CAD build for the part. Positions are in the model's coordinates, mm. Round coordinates to 2 decimals unless told otherwise and drop trailing zeros. Loops run counter-clockwise (first coordinate to the right, second up) from the corner with the lowest first, then second, coordinate; pieces in that order, holes last. Notation, with made-up numbers: M -38,57.25 L 12,57.25 A23 ccw 12,89.25 Z; hole C 12,51 d10. An arc over 180 degrees is marked long. Put each result on its own line as item: value. Start each with the question number.
from build123d import *

# Parameters (mm, degrees)
F0_R     = 2.725
F0_R_2   = 10
F0_R_3   = 1
F1_DEPTH = 1.8
F2_DEPTH = 6.3
F3_DEPTH = 6.3
F4_DEPTH = 6.25


with BuildPart() as f1:
    # F0 (on Top) → F1 (new body)
    with BuildSketch(Plane.XY):
        with BuildLine():
            Line((38.875, -34.725), (38.875, 34.725))
            ThreePointArc((38.875, 34.725), (37.659493, 37.659493), (34.725, 38.875))
            Line((34.725, 38.875), (-34.725, 38.875))
            ThreePointArc((-34.725, 38.875), (-37.659493, 37.659493), (-38.875, 34.725))
            Line((-38.875, 34.725), (-38.875, -34.725))
            ThreePointArc((-38.875, -34.725), (-37.659493, -37.659493), (-34.725, -38.875))
            Line((-34.725, -38.875), (34.725, -38.875))
            ThreePointArc((34.725, -38.875), (37.659493, -37.659493), (38.875, -34.725))
        make_face()
        with Locations((-22.925, -34.725)):
            Circle(F0_R, mode=Mode.SUBTRACT)
        with Locations((22.925, -34.725)):
            Circle(F0_R, mode=Mode.SUBTRACT)
        with Locations((-22.925, 34.725)):
            Circle(F0_R, mode=Mode.SUBTRACT)
        Circle(F0_R_2, mode=Mode.SUBTRACT)
        with Locations((22.925, 34.725)):
            Circle(F0_R, mode=Mode.SUBTRACT)
        with Locations((-22.925, 34.725)):
            Circle(F0_R)
        with Locations((-22.925, 34.725)):
            Circle(F0_R_3, mode=Mode.SUBTRACT)
        with Locations((-22.925, 34.725)):
            Circle(F0_R_3)
        with Locations((22.925, -34.725)):
            Circle(F0_R)
        with Locations((22.925, -34.725)):
            Circle(F0_R_3, mode=Mode.SUBTRACT)
        with Locations((22.925, -34.725)):
            Circle(F0_R_3)
        with Locations((-22.925, -34.725)):
            Circle(F0_R)
        with Locations((-22.925, -34.725)):
            Circle(F0_R_3, mode=Mode.SUBTRACT)
        with Locations((-22.925, -34.725)):
            Circle(F0_R_3)
        with Locations((22.925, 34.725)):
            Circle(F0_R)
        with Locations((22.925, 34.725)):
            Circle(F0_R_3, mode=Mode.SUBTRACT)
        with Locations((22.925, 34.725)):
            Circle(F0_R_3)
    extrude(amount=F1_DEPTH)

    # F0 (on Top) → F2 (join)
    with BuildSketch(Plane.XY):
        with BuildLine():
            Line((-34.725, -40.725), (34.725, -40.725))
            ThreePointArc((34.725, -40.725), (38.967641, -38.967641), (40.725, -34.725))
            Line((40.725, -34.725), (40.725, 34.725))
            ThreePointArc((40.725, 34.725), (38.967641, 38.967641), (34.725, 40.725))
            Line((34.725, 40.725), (-34.725, 40.725))
            ThreePointArc((-34.725, 40.725), (-38.967641, 38.967641), (-40.725, 34.725))
            Line((-40.725, 34.725), (-40.725, -34.725))
            ThreePointArc((-40.725, -34.725), (-38.967641, -38.967641), (-34.725, -40.725))
        make_face()
        with BuildLine():
            ThreePointArc((34.725, 38.875), (37.659493, 37.659493), (38.875, 34.725))
            Line((38.875, 34.725), (38.875, -34.725))
            ThreePointArc((38.875, -34.725), (37.659493, -37.659493), (34.725, -38.875))
            Line((34.725, -38.875), (-34.725, -38.875))
            ThreePointArc((-34.725, -38.875), (-37.659493, -37.659493), (-38.875, -34.725))
            Line((-38.875, -34.725), (-38.875, 34.725))
            ThreePointArc((-38.875, 34.725), (-37.659493, 37.659493), (-34.725, 38.875))
            Line((-34.725, 38.875), (34.725, 38.875))
        make_face(mode=Mode.SUBTRACT)
    extrude(amount=F2_DEPTH)

    # F0 (on Top) → F3 (join)
    with BuildSketch(Plane.XY):
        with Locations((-22.925, 34.725)):
            Circle(F0_R)
        with Locations((-22.925, 34.725)):
            Circle(F0_R_3, mode=Mode.SUBTRACT)
    extrude(amount=F3_DEPTH)

    # F0 (on Top) → F4 (join)
    with BuildSketch(Plane.XY):
        with Locations((22.925, 34.725)):
            Circle(F0_R)
        with Locations((22.925, 34.725)):
            Circle(F0_R_3, mode=Mode.SUBTRACT)
        with Locations((22.925, -34.725)):
            Circle(F0_R)
        with Locations((22.925, -34.725)):
            Circle(F0_R_3, mode=Mode.SUBTRACT)
        with Locations((-22.925, -34.725)):
            Circle(F0_R)
        with Locations((-22.925, -34.725)):
            Circle(F0_R_3, mode=Mode.SUBTRACT)
    extrude(amount=F4_DEPTH)


solid = f1.part
(1) Cut at A-A on z = 3.5. Count the separate pieces of the cut face and the enclosed holes in it, and give its area (3 significant figures).
(2) Mould opens along Y. For faces 1 (the cylindrical face through (-23.662, 35.401, 4.018)), 2 (the cylindrical face through (-38.921, 39.014, 3.106)), 3 (the flat face through (40.725, 0, 3)) say: +Y half, -Y half, draft (parallel to the pull), parting line (faces both ways), or undercut.
(3) Drill centre lines: line 1 along Y through (x, z) = (23, 6) (3 decimals); line 2 along Y through (x, z) = (14, 6) (3 decimals). Where is each one in solid material? Low to high.
(4) Cut at D-D on x = 27. List the corners of the cut face in (y, z) (3 decimals).
(5) Cut at B-B on y = 0. List the corners of the cut face in (x, z) (3 decimals), and give its area (3 significant figures).
(6) Flat gauge pins, fed straight in: pin 1 Ø2 at (x, y) = (23, -34.5) entering from +Z; pin 2 Ø1.6 at (x, y) = (22.925, 34.725) entering from +Z. Where does each tip first touch, or does it go through?
Taken from the geometry:
1. separate pieces: 5
1. enclosed holes: 5
1. area: 654 mm2
2. face 1: undercut
2. face 2: +Y half
2. face 3: draft
3. line 1: -40.725 to -38.875, -37.449 to -35.722, -33.728 to -32.001, 32.001 to 33.728, 35.722 to 37.449, 38.875 to 40.725
3. line 2: -40.725 to -38.875, 38.875 to 40.725
4. outline: M -40.725,0 L 40.725,0 L 40.725,6.3 L 38.875,6.3 L 38.875,1.8 L -38.875,1.8 L -38.875,6.3 L -40.725,6.3 Z
5. outline: M -40.725,0 L -10,0 L -10,1.8 L -38.875,1.8 L -38.875,6.3 L -40.725,6.3 Z; M 10,0 L 40.725,0 L 40.725,6.3 L 38.875,6.3 L 38.875,1.8 L 10,1.8 Z
5. area: 127 mm2
6. pin 1: z = 6.25
6. pin 2: z = 1.8
